from build123d import *

# Parameters (mm, degrees)
SKETCH1_R           = 47.5
BOSS_EXTRUDE2_DEPTH = 25
FILLET1_R           = 20
SKETCH3_R           = 10
BOSS_EXTRUDE3_DEPTH = 5
SKETCH4_R           = 27.5
CUT_EXTRUDE1_DEPTH  = 7.5
SKETCH5_R           = 10
BOSS_EXTRUDE5_DEPTH = 7.5
SKETCH6_W           = 48.682304138
SKETCH6_H           = 105.772137124
CUT_EXTRUDE2_DEPTH  = 50
SCALE4_SCALE        = 1.15


with BuildPart() as part:
    # Sketch1 → Boss-Extrude2 (new body)
    with BuildSketch(Plane.XY):
        Circle(SKETCH1_R)
    extrude(amount=BOSS_EXTRUDE2_DEPTH)

    # Fillet1
    fillet1_edges = [part.edges().sort_by_distance(p)[0] for p in [
        (-47.5, 0, 25),
    ]]
    fillet(fillet1_edges, radius=FILLET1_R)

    # Sketch3 → Boss-Extrude3 (add)
    with BuildSketch(Plane.XY.offset(25)):
        Circle(SKETCH3_R)
    extrude(amount=-BOSS_EXTRUDE3_DEPTH)

    # Sketch4 → Cut-Extrude1 (cut)
    with BuildSketch(Plane.XY.offset(25)):
        Circle(SKETCH4_R)
    extrude(amount=-CUT_EXTRUDE1_DEPTH, mode=Mode.SUBTRACT)

    # Sketch5 → Boss-Extrude5 (add)
    with BuildSketch(Plane.XY.offset(17.5)):
        Circle(SKETCH5_R)
    extrude(amount=BOSS_EXTRUDE5_DEPTH)

    # Sketch6 → Cut-Extrude2 (cut)
    with BuildSketch(Plane.XY.offset(25)):
        with Locations((-24.341152069, -1.830671604)):
            Rectangle(SKETCH6_W, SKETCH6_H)
    extrude(amount=-CUT_EXTRUDE2_DEPTH, mode=Mode.SUBTRACT)


with BuildPart() as part_1:
    # Scale4: scaled about (19.733587982, 0, 10.209783997)
    add(part.part.scale(SCALE4_SCALE).moved(Location((-2.960038197, 0, -1.5314676))))


solid = part_1.part
Could you check a few things on this model? Use its own coordinates, in mm. A direction names the side the tool comes from. Give positions to 0.01 mm unless a question says otherwise; leave off trailing zeros. Loops run counter-clockwise (first coordinate to the right, second up) from the corner with the lowest first, then second, coordinate; pieces in that order, holes last. Notation, with made-up numbers: (-34, 34) -> (-27, 34) arc R13 cw to (-27, 52) -> close; hole circle Ø7 at (-8, 39). An arc over 180 degrees is marked (long way). Return JSON: item names as keys, results as strings.
Item 1: If we section it at A-A on y = 0: List the corners of the cut face in (x, z) for me, plus the area to 3 significant figures.
Geometry results:
{"outline": "(-2.96, -1.53) -> (51.66, -1.53) -> (51.66, 4.22) arc R23 ccw to (28.66, 27.22) -> (28.66, 18.59) -> (8.54, 18.59) -> (8.54, 27.22) -> (-2.96, 27.22) -> close", "area": "1,280 mm²"}
Item 2: I need wall thicknesses on L1, parallel to Z at x = 27, y = 3; L2, parallel to Y at x = 16, z = 15.25; L3, parallel to Y at x = 12.5, z = 24.75. Which ranges of each line are inside material? Lowest first, please. Write a range as from..to.
Geometry results:
{"L1": "z = -1.53..18.59", "L2": "y = -48.21..48.21", "L3": "y = -39.04..-27.59, 27.59..39.04"}
Item 3: We'd pull the mould along Y, two halves only. Please class faces 3 (the cylindrical face through (28.657, -0.695, 22.966)), 4 (the flat face through (18, 1, -1.531)), 5 (the cylindrical face through (8.537, -0.253, 22.846)), 6 (the cylindrical face through (51.65, -1.2, 1.3)): +Y half, -Y half, draft (parallel to the pull), parting line (faces both ways), or undercut.
Geometry results:
{"face 3": "undercut", "face 4": "draft", "face 5": "undercut", "face 6": "parting line"}
Item 4: If we section it at C-C on z = 7.25: List the corners of the cut face in (x, y) for me.
Geometry results:
{"outline": "(-2.96, -54.42) arc R54.42 ccw to (-2.96, 54.42) -> close"}
Item 5: Which directions (+Z, -Z, +X, -X, +Y, -Y) give clear straight access to the entire face, cutting with the end or side of a thin tool? Please do faces 1 (the flat face through (13, 0, 18.594)), 2 (the flat face through (-2.96, -1, 10)).
Geometry results:
{"face 1": "+Z", "face 2": "+Z, -Z, -X, +Y, -Y"}
Item 6: If we section it at B-B on z = 15: List the corners of the cut face in (x, y) for me, plus the area to 3 significant figures.
Geometry results:
{"outline": "(-2.96, -51.94) arc R51.94 ccw to (-2.96, 51.94) -> close", "area": "4,240 mm²"}
Item 7: I'm going to push flat-ended pins straight in: pin 1 (1 mm diameter, centred on x = 19.5, y = -19.5, fed in from +Z); pin 2 (16 mm diameter, centred on x = 13.5, y = 5, fed in from +Z); pin 3 (4 mm diameter, centred on x = 26.5, y = -40, fed in from +Z); pin 4 (6 mm diameter, centred on x = 23.5, z = 23.5, fed in from -Y). Where does each tip first touch, or does it pass through?
Geometry results:
{"pin 1": "stops at z = 18.59", "pin 2": "stops at z = 27.22", "pin 3": "stops at z = 20.69", "pin 4": "stops at y = -40.37"}
